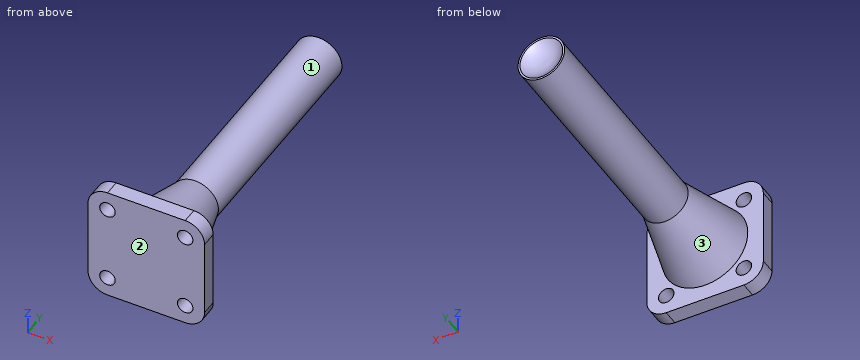
```python
from build123d import *

# Parameters (mm, degrees)
SKETCH_1_W      = 30
SKETCH_1_H      = 30
SKETCH_1_R      = 2
EXTRUDE_1_DEPTH = 4
FILLET_1_R      = 5
SKETCH_2_R      = 6
EXTRUDE_2_DEPTH = 76
CHAMFER_1_SIZE  = 5
CHAMFER_1_SIZE2 = 18.660254038


with BuildPart() as part:
    # Эскиз1 → Бобышка-Вытянуть1 (new body)
    with BuildSketch(Plane(origin=(0, 0, 0), x_dir=(1, 0, 0), z_dir=(0, 1, 0))):
        Rectangle(SKETCH_1_W, SKETCH_1_H)
        with Locations(Location((-10, 10, 0), (0, 0, 270))):
            Circle(SKETCH_1_R, mode=Mode.SUBTRACT)
        with Locations(Location((10, 10, 0), (0, 0, 270))):
            Circle(SKETCH_1_R, mode=Mode.SUBTRACT)
        with Locations(Location((10, -10, 0), (0, 0, 270))):
            Circle(SKETCH_1_R, mode=Mode.SUBTRACT)
        with Locations(Location((-10, -10, 0), (0, 0, 270))):
            Circle(SKETCH_1_R, mode=Mode.SUBTRACT)
    extrude(amount=EXTRUDE_1_DEPTH)

    # Скругление1
    fillet_1_edges = [part.edges().sort_by_distance(p)[0] for p in [
        (15, 2, 15),
        (-15, 2, 15),
        (-15, 2, -15),
        (15, 2, -15),
    ]]
    fillet(fillet_1_edges, radius=FILLET_1_R)

    # Эскиз2 → Бобышка-Вытянуть2 (add)
    with BuildSketch(Plane(origin=(0, 4, 0), x_dir=(1, 0, 0), z_dir=(0, 1, 0))):
        with Locations(Location((0, 0, 0), (0, 0, 270))):
            Circle(SKETCH_2_R)
    extrude(amount=EXTRUDE_2_DEPTH)

    # Эскиз7 → Вырез-Повернуть3 (revolve, cut)
    with BuildSketch(Plane.XY):
        with BuildLine():
            Line((5.5, 80), (0, 80))
            Line((0, 80), (0, 78))
            ThreePointArc((0, 78), (2.979435889, 78.369051304), (5.5, 80))
        make_face()
    revolve(axis=Axis((0, 82.404747685, 0), (0, -1, 0)), mode=Mode.SUBTRACT)

    # Фаска1
    chamfer_1_edges = [part.edges().sort_by_distance(p)[0] for p in [
        (0, 4, -6),
    ]]
    chamfer_1_side = [part.faces().sort_by_distance(p)[0] for p in [
        (0, 4, 14.575735931),
    ]]
    chamfer(chamfer_1_edges, length=CHAMFER_1_SIZE, length2=CHAMFER_1_SIZE2, reference=chamfer_1_side[0])


solid = part.part
```
Model file for the job. Use its own axes, mm. Face numbers are marked on the shaded views. Coordinates: 2 decimals unless noted, no trailing zeros. Loops run counter-clockwise (first coordinate to the right, second up) from the corner with the lowest first, then second, coordinate; pieces in that order, holes last. Notation, with made-up numbers: (-6, 26.5) - (8, 26.5) arc R25 cw to (8, 39.5) - close; hole circle Ø8 at (59.5, 64). An arc over 180 degrees is marked (long way). Write item = value, one per line. Start each with the question number.
Item 1: Saw through at B-B, the plane z = 9. State how many separate pieces and enclosed holes the cut face has, then the cut area to 3 significant figures.
Item 2: Drop flat-ended pins along their axis: pin 1 Ø12 at (y, z) = (22.5, -2.5) entering from +X; pin 2 Ø9 at (x, z) = (2.5, -1.5) entering from +Y; pin 3 Ø1.5 at (y, z) = (17, 10) entering from +X; pin 4 Ø2 at (y, z) = (44, 0.5) entering from -X. Give the stop position or say it passes through.
Item 3: Saw through at C-C, the plane y = 19. List the corners of the cut face in (x, z), then the cut area to 3 significant figures.
Item 4: Saw through at A-A, the plane y = 30. List the corners of the cut face in (x, z), then the cut area to 3 significant figures.
Item 5: Pull direction Y, two halves, no side cores. Call the marked faces 1, 2 and 3: +Y half, -Y half, draft (parallel to the pull), parting line (faces both ways), or undercut.
Item 6: Wall check: probe 1 along X at (y, z) = (2.1, -10); probe 2 along Y at (x, z) = (12.75, -8.25); probe 3 along Z at (x, y) = (-0.25, 43). Give the ranges that are in metal, low to high. Write a range as [from, to].
Answers:
q1.separate_pieces = 3
q1.enclosed_holes = 0
q1.area = 154 mm2
q2.pin_1 = 7.54
q2.pin_2 = 80
q2.pin_3 = through
q2.pin_4 = -6
q3.outline = circle Ø13.96 at (0, 0)
q3.area = 153 mm2
q4.outline = circle Ø12 at (0, 0)
q4.area = 113 mm2
q5.face_1 = draft
q5.face_2 = -Y half
q5.face_3 = +Y half
q6.probe_1 = [-15, -12], [-8, 8], [12, 15]
q6.probe_2 = [0, 4]
q6.probe_3 = [-5.99, 5.99]
